CAD build for the part. Positions are in the model's coordinates, mm. A direction names the side the tool comes from. Give positions to 0.01 mm unless a question says otherwise; leave off trailing zeros. Loops run counter-clockwise (first coordinate to the right, second up) from the corner with the lowest first, then second, coordinate; pieces in that order, holes last. Notation, with made-up numbers: M -17.5,74 L 32.5,74 A24 ccw 32.5,113 Z; hole C 40,89.5 d11. An arc over 180 degrees is marked long. One line per question, with ' | ' between items.
```python
from build123d import *

# Parameters (mm, degrees)
SKETCH_3_W                                  = 24
SKETCH_3_H                                  = 16
V10_TOF_CANDIDATE_CARRIER24X16_DEPTH        = 1.6
V10_TOF_OPTICAL_PACKAGES_FACING_FRONT_START = 1.6
SKETCH_4_R                                  = 1.3
V10_TOF_OPTICAL_PACKAGES_FACING_FRONT_DEPTH = 1.4
SKETCH_5_R                                  = 1.3
V10_TOF_TWO_CANDIDATE_HOLES20MM_DEPTH       = 1.6


with BuildPart() as part:
    # 草图3 → V10_TOF_candidate_carrier24x16 (new body)
    with BuildSketch(Plane.XY):
        with Locations((0, 88)):
            Rectangle(SKETCH_3_W, SKETCH_3_H)
    extrude(amount=V10_TOF_CANDIDATE_CARRIER24X16_DEPTH)

    # 草图4 → V10_TOF_optical_packages_facing_front (add)
    with BuildSketch(Plane.XY.offset(V10_TOF_OPTICAL_PACKAGES_FACING_FRONT_START)):
        with Locations((-1.6, 88)):
            Circle(SKETCH_4_R)
        with Locations((1.6, 88)):
            Circle(SKETCH_4_R)
    extrude(amount=V10_TOF_OPTICAL_PACKAGES_FACING_FRONT_DEPTH)

    # 草图5 → V10_TOF_two_candidate_holes20mm (cut)
    with BuildSketch(Plane.XY.offset(1.6)):
        with Locations((-10, 82)):
            Circle(SKETCH_5_R)
        with Locations((10, 82)):
            Circle(SKETCH_5_R)
    extrude(amount=-V10_TOF_TWO_CANDIDATE_HOLES20MM_DEPTH, mode=Mode.SUBTRACT)


solid = part.part
```
Item 1: Drill centre lines: line 1 along X through (y, z) = (82, 0.6); line 2 along Y through (x, z) = (10, 0.65); line 3 along Z through (x, y) = (0.75, 86.5). Where is each one in solid material? Low to high. Write a range as [from, to].
Conclusion:
line 1: [-12, -11.3], [-8.7, 8.7], [11.3, 12] | line 2: [80, 80.7], [83.3, 96] | line 3: [0, 1.6]
Item 2: Drop a flat-ended pin along its axis: P1, Ø2, axis at x = 5, y = 88.5, coming from the +Z side. Give the stop position or say it passes through.
Conclusion:
P1: z = 1.6
Item 3: Saw through at D-D on y = 88. Give the cut face in (x, z).
Conclusion:
outline: M -12,0 L 12,0 L 12,1.6 L 2.9,1.6 L 2.9,3 L 0.3,3 L 0.3,1.6 L -0.3,1.6 L -0.3,3 L -2.9,3 L -2.9,1.6 L -12,1.6 Z
Item 4: Saw through at B-B on x = 10. Give the cut face in (y, z), and give its area (3 significant figures).
Conclusion:
outline: M 80,0 L 80.7,0 L 80.7,1.6 L 80,1.6 Z; M 83.3,0 L 96,0 L 96,1.6 L 83.3,1.6 Z | area: 21.4 mm²
Item 5: 3-axis set-ups, long thin cutter, end or side, ignore diameter. For faces 5 (the cylindrical face through (1.32, 86.73, 2.29)), 6 (the flat face through (0, 88, 0)): which of +Z, -Z, +X, -X, +Y, -Y reach the whole face in a straight line?
Conclusion:
face 5: +Z | face 6: -Z, +X, -X, +Y, -Y
Item 6: Saw through at C-C on z = 0.45. Give the cut face in (x, y), and give its area (3 significant figures).
Conclusion:
outline: M -12,80 L 12,80 L 12,96 L -12,96 Z; hole C -10,82 d2.6; hole C 10,82 d2.6 | area: 373 mm²
Item 7: Saw through at A-A on y = 82. Give the cut face in (x, z), and give its area (3 significant figures).
Conclusion:
outline: M -12,0 L -11.3,0 L -11.3,1.6 L -12,1.6 Z; M -8.7,0 L 8.7,0 L 8.7,1.6 L -8.7,1.6 Z; M 11.3,0 L 12,0 L 12,1.6 L 11.3,1.6 Z | area: 30.1 mm²
Item 8: Mould opens along X. For faces 1 (the flat face through (-12, 88, 1)), 2 (the flat face through (0, 96, 1)), 3 (the cylindrical face through (-10.28, 80.73, 0.81)), 4 (the cylindrical face through (9.72, 80.73, 0.81)) say: pulls with the +X half, pulls with the -X half, needs draft (parallel to the pull), parting line crosses it, or undercut.
Conclusion:
face 1: pulls with the -X half | face 2: needs draft | face 3: undercut | face 4: undercut
